Model file for the job. Use its own axes, mm. Face numbers are marked on the shaded views. A direction names the side the tool comes from. Give positions to 0.01 mm unless a question says otherwise; leave off trailing zeros. Write each loop counter-clockwise with the first axis right and the second up, starting at its lowest first coordinate (ties: lowest second). Pieces come first, ordered by that corner, then holes. Notation, with made-up numbers: (-10.75, 87.5) - (47.25, 87.5) arc R27 cw to (47.25, 126.5) - close; hole circle Ø4 at (-7.5, 81). An arc over 180 degrees is marked (long way). One line per item, written item: value. Start each with the question number.
(1) Cut at D-D, the plane z = 18. List the corners of the cut face in (x, y).
(2) Cut at B-B, the plane y = -41. List the corners of the cut face in (x, z).
(3) Probe L1, parallel to X at y = -29, z = 0; L2, parallel to Z at x = -11, y = -21.5; L3, parallel to X at y = -37, z = 3.5. List the from-to ranges inside material, lowest first.
(4) Cut at A-A, the plane z = 49. List the corners of the cut face in (x, y), and give its area (3 significant figures).
(5) Drop flat-ended pins along their axis: P1, Ø1, axis at y = -32.5, z = 84.5, coming from the -X side; P2, Ø1, axis at x = 74, z = 83.5, coming from the +Y side; P3, Ø2, axis at x = 82.5, y = -15.5, coming from the -Z side. Give the stop position or say it passes through.
(6) Cut at C-C, the plane x = 27.5. List the corners of the cut face in (y, z).
(7) 3-axis set-ups, long thin cutter, end or side, ignore diameter. For the marked faces 1, 2 and 3: which of +Z, -Z, +X, -X, +Y, -Y reach the whole face in a straight line?
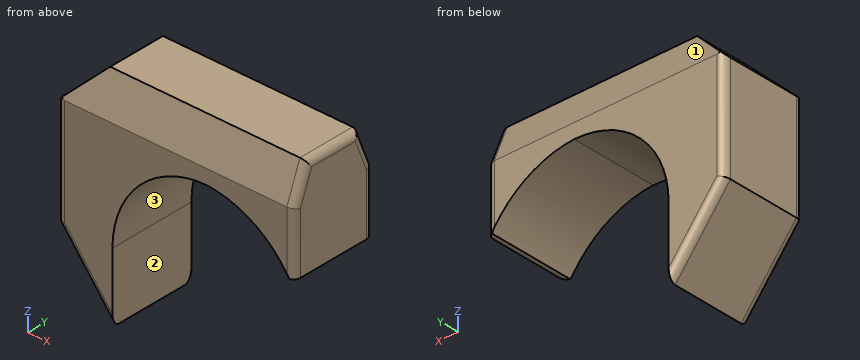
from build123d import *

# Parameters (mm, degrees)
F1_DEPTH = 60
F2_SIZE2 = 25
F2_SIZE  = 10
F3_R     = 5


with BuildPart() as f1:
    # F0 (on Front) → F1 (new body)
    with BuildSketch(Plane.XZ):
        with BuildLine():
            Line((125, 32.1942828596), (125, 75))
            Line((125, 75), (125, 100))
            Line((125, 100), (-10.5827422813, 100))
            Line((-10.5827422813, 100), (-38.1556677818, 73.0981135368))
            Line((-38.1556677818, 73.0981135368), (-38.1556677818, 0))
            Line((-38.1556677818, 0), (0, -47.6187802851))
            Line((0, -47.6187802851), (0, 0))
            ThreePointArc((0, 0), (19.0380592229, 45.9619407771), (65, 65))
            ThreePointArc((65, 65), (97.417599338, 55.5490608419), (121.8056157231, 32.1942828596))
            Line((121.8056157231, 32.1942828596), (125, 32.1942828596))
        make_face()
    extrude(amount=F1_DEPTH)

    # F2
    f2_edges = [f1.edges().sort_by_distance(p)[0] for p in [
        (57.208629, -60, 100),
        (57.208629, 0, 100),
    ]]
    f2_side = f1.faces().sort_by_distance((57.208629, -30, 100))[0]
    chamfer(f2_edges, length=F2_SIZE, length2=F2_SIZE2, reference=f2_side)

    # F3
    f3_edges = [f1.edges().sort_by_distance(p)[0] for p in [
        (125, -30, 100),
        (125, -60, 53.597141),
        (125, 0, 53.597141),
        (-38.155668, -60, 36.549057),
        (-38.155668, 0, 36.549057),
        (-19.077834, 0, -23.80939),
        (-19.077834, -60, -23.80939),
        (125, -5, 87.5),
        (125, -55, 87.5),
    ]]
    fillet(f3_edges, radius=F3_R)


solid = f1.part
Answers follow:
1. outline: (-38.16, -55) arc R5 ccw to (-33.16, -60) - (2.54, -60) - (2.54, 0) - (-33.16, 0) arc R5 ccw to (-38.16, -5) - close
2. outline: (-38.16, 0) - (0, -47.62) - (0, 0) arc R65 cw to (65, 65) arc R71.02 cw to (121.81, 32.19) - (125, 32.19) - (125, 95) arc R5 ccw to (120, 100) - (-10.58, 100) - (-38.16, 73.1) - close
3. L1: x = -38.16 to 0
3. L2: z = -33.89 to 99.59
3. L3: x = -38.16 to 0.09
4. outline: (-38.16, -55) arc R5 ccw to (-33.16, -60) - (22.29, -60) - (22.29, 0) - (-33.16, 0) arc R5 ccw to (-38.16, -5) - close; (106.89, -60) - (120, -60) arc R5 ccw to (125, -55) - (125, -5) arc R5 ccw to (120, 0) - (106.89, 0) - close
4. area: 4,690 mm²
5. P1: stops at x = -26.98
5. P2: stops at y = -3.2
5. P3: stops at z = 61.7
6. outline: (-60, 53.09) - (0, 53.09) - (0, 75) - (-10, 100) - (-50, 100) - (-60, 75) - close
7. face 1: +Z, +X, -X, +Y
7. face 2: -Z, +X, +Y, -Y
7. face 3: -Z, +Y, -Y
